Build history of the part. All positions in model axes, mm. A direction names the side the tool comes from. Give positions to 0.01 mm unless a question says otherwise; leave off trailing zeros. Order: outer loops, then holes, each group sorted by start corner. A loop starts at its lowest first (then second) coordinate and runs counter-clockwise, first axis right, second up. Notation, with made-up numbers: (17.25, 87.25) -> (55.25, 87.25) arc R28 cw to (55.25, 124.25) -> close; hole circle Ø8 at (22, 29). An arc over 180 degrees is marked (long way). One line per question, with ' | ' between items. Start each with the question number.
(1) Cut at D-D (z = -2). Give the cut face in (x, y) (3 decimals), then the cut area to 3 significant figures.
(2) Pin check, flat tips, straight feed: pin 1 Ø3 at (x, z) = (20.5, -3.5) entering from +Y; pin 2 Ø3 at (x, z) = (-23.5, -0.5) entering from +Y; pin 3 Ø1.5 at (x, z) = (-26.5, 2) entering from +Y. Stop position of each tip, or through.
(3) Cut at A-A (y = 0). Give the cut face in (x, z) (3 decimals).
(4) Cut at C-C (z = 15). Give the cut face in (x, y), then the cut area to 3 significant figures.
(5) Which spindle directions (+Z, -Z, +X, -X, +Y, -Y) get a long thin tool onto all of the face, cutting with end or side? Do faces 1 (the face through (-13, 36, 0)), 2 (the face through (-5.175, 39.412, 16.93)), 3 (the face through (28, 45, 10)). Say none if no direction does.
(6) Drill centre lines: L1, parallel to Y at x = 0, z = 15; L2, parallel to X at y = -7, z = 14.5; L3, parallel to Y at x = 0, z = 9. Where is each one in solid material? Low to high. Write a range as from..to.
from build123d import *

# Parameters (mm, degrees)
F0_R     = 53
F0_R_2   = 50.25
F1_DEPTH = 22
F0_R_3   = 39.75
F0_R_4   = 17.5
F2_SIZE  = 1
F3_DEPTH = 12
F4_R     = 37.625
F4_R_2   = 17.5
F5_DEPTH = 9
F6_SIZE  = 2


with BuildPart() as f1:
    # F0 (on Top) → F1 (new body)
    with BuildSketch(Plane.XY):
        Circle(F0_R)
        Circle(F0_R_2, mode=Mode.SUBTRACT)
    extrude(amount=F1_DEPTH)

    # F2
    f2_edges = [f1.edges().sort_by_distance(p)[0] for p in [
        (-53, 0, 22),
    ]]
    chamfer(f2_edges, length=F2_SIZE)



with BuildPart() as f1b:
    # F0 (on Top) → F1, piece 2 (new body)
    with BuildSketch(Plane.XY):
        Circle(F0_R_3)
        Circle(F0_R_4, mode=Mode.SUBTRACT)
    extrude(amount=F1_DEPTH)


with BuildPart() as f1_1:
    add(f1.part)

    add(f1b.part)  # F3 merges F1b
    # F0 (on Top) → F3 (join)
    with BuildSketch(Plane.XY):
        Circle(F0_R_2)
        Circle(F0_R_3, mode=Mode.SUBTRACT)
    extrude(amount=F3_DEPTH)

    # F4 (on face) → F5 (join)
    with BuildSketch(Plane.XY):
        Circle(F4_R)
        Circle(F4_R_2, mode=Mode.SUBTRACT)
    extrude(amount=-F5_DEPTH)

    # F6
    f6_edges = [f1_1.edges().sort_by_distance(p)[0] for p in [
        (-37.625, 0, -9),
    ]]
    chamfer(f6_edges, length=F6_SIZE)


solid = f1_1.part
Result set:
1) outline: circle Ø75.25 at (0, 0); hole circle Ø35 at (0, 0) | area: 3,490 mm2
2) pin 1: stops at y = 32.48 | pin 2: stops at y = 48.18 | pin 3: stops at y = 46.32
3) outline: (-53, 0) -> (-37.625, 0) -> (-37.625, -7) -> (-35.625, -9) -> (-17.5, -9) -> (-17.5, 22) -> (-39.75, 22) -> (-39.75, 12) -> (-50.25, 12) -> (-50.25, 22) -> (-52, 22) -> (-53, 21) -> close; (17.5, -9) -> (35.625, -9) -> (37.625, -7) -> (37.625, 0) -> (53, 0) -> (53, 21) -> (52, 22) -> (50.25, 22) -> (50.25, 12) -> (39.75, 12) -> (39.75, 22) -> (17.5, 22) -> close
4) outline: circle Ø106 at (0, 0); circle Ø79.5 at (0, 0); hole circle Ø100.5 at (0, 0); hole circle Ø35 at (0, 0) | area: 4,890 mm2
5) face 1: -Z | face 2: +Z | face 3: +Z, -Z
6) L1: y = -53..-50.25, -39.75..-17.5, 17.5..39.75, 50.25..53 | L2: x = -52.54..-49.76, -39.13..-16.04, 16.04..39.13, 49.76..52.54 | L3: y = -53..-17.5, 17.5..53
